Here's how the part is built. I have some questions about the finished solid (model axes, mm). A direction names the side the tool comes from. Round coordinates to 2 decimals unless told otherwise and drop trailing zeros. Order: outer loops, then holes, each group sorted by start corner. A loop starts at its lowest first (then second) coordinate and runs counter-clockwise, first axis right, second up.
```python
from build123d import *

# Parameters (mm, degrees)
F1_DEPTH = 15
F2_W     = 81.2403840464
F2_H     = 7.5
F3_DEPTH = 15
F4_DEPTH = 0.62
F5_DEPTH = 0.62


with BuildPart() as f1:
    # F0 (on Top) → F1 (new body)
    with BuildSketch(Plane.XY):
        with BuildLine():
            Line((-8.2947787642, 47.5), (-8.2947787642, 0))
            Line((-8.2947787642, 0), (20.2052212358, 0))
            ThreePointArc((20.2052212358, 0), (26.7052212358, 6.5), (33.2052212358, 0))
            Line((33.2052212358, 0), (54.2052212358, 0))
            ThreePointArc((54.2052212358, 0), (48.4723420076, 26.148498987), (32.3254132589, 47.5))
            Line((32.3254132589, 47.5), (-8.2947787642, 47.5))
        make_face()
        with BuildLine():
            Line((20.2052212358, 0), (-8.2947787642, 0))
            Line((-8.2947787642, 0), (-8.2947787642, -62.5))
            ThreePointArc((-8.2947787642, -62.5), (35.8993950599, -44.1941738242), (54.2052212358, 0))
            Line((54.2052212358, 0), (33.2052212358, 0))
            ThreePointArc((33.2052212358, 0), (26.7052212358, -6.5), (20.2052212358, 0))
        make_face()
        with BuildLine():
            Line((-8.2947787642, 0), (-36.7947787642, 0))
            ThreePointArc((-36.7947787642, 0), (-43.2947787642, -6.5), (-49.7947787642, 0))
            Line((-49.7947787642, 0), (-70.7947787642, 0))
            ThreePointArc((-70.7947787642, 0), (-52.4889525884, -44.1941738242), (-8.2947787642, -62.5))
            Line((-8.2947787642, -62.5), (-8.2947787642, 0))
        make_face()
        with BuildLine():
            ThreePointArc((-49.7947787642, 0), (-43.2947787642, 6.5), (-36.7947787642, 0))
            Line((-36.7947787642, 0), (-8.2947787642, 0))
            Line((-8.2947787642, 0), (-8.2947787642, 47.5))
            Line((-8.2947787642, 47.5), (-48.9149707874, 47.5))
            ThreePointArc((-48.9149707874, 47.5), (-65.0618995361, 26.148498987), (-70.7947787642, 0))
            Line((-70.7947787642, 0), (-49.7947787642, 0))
        make_face()
    extrude(amount=F1_DEPTH)

    # F2 (on face) → F3 (cut)
    with BuildSketch(Plane(origin=(0, 47.5, 0), x_dir=(-1, 0, 0), z_dir=(0, 1, 0))):
        with Locations((8.2947787642, 3.75)):
            Rectangle(F2_W, F2_H)
    extrude(amount=-F3_DEPTH, mode=Mode.SUBTRACT)

    # F4 (add): a face of the model
    f4_faces = [f1.faces().sort_by_distance(p)[0] for p in [
        (-48.9149707874, 40, 3.75),
    ]]
    extrude(f4_faces, amount=F4_DEPTH)

    # F5 (add): a face of the model
    f5_faces = [f1.faces().sort_by_distance(p)[0] for p in [
        (32.3254132589, 40, 3.75),
    ]]
    extrude(f5_faces, amount=F5_DEPTH)


solid = f1.part
```
1) For faces 1 (the flat face through (-7, -7, 0)), 2 (the flat face through (-48.295, 40, 4)), which set-ups out of +Z, -Z, +X, -X, +Y, -Y let a thin tool reach every point of the face, with its end or its side?
2) If we section it at C-C (x = 12): Write out the boundary of the cut face in (y, z), plus the area to 3 significant figures.
3) If we section it at D-D (z = 4): Write out the boundary of the cut face in (x, y).
4) If we section it at B-B (y = -3.5): Write out the boundary of the cut face in (x, z).
5) I'm going to push flat-ended pins straight in: pin 1 (16.5 mm diameter, centred on x = -0.5, y = 41.5, fed in from -Z); pin 2 (1.5 mm diameter, centred on y = 11.5, z = 3.5, fed in from -X); pin 3 (11.5 mm diameter, centred on x = -43.29, y = 0, fed in from +Z); pin 4 (2 mm diameter, centred on y = -50.5, z = 2, fed in from +X). Where does each tip first touch, or does it pass through?
6) We'd pull the mould along X, two halves only. Please class faces 3 (the flat face through (-8, 32.5, 4)), 4 (the flat face through (-8, 47.5, 12)): +X half, -X half, draft (parallel to the pull), parting line (faces both ways), or undercut.
7) I need wall thicknesses on line 1 (Y direction, x = 27, z = 14); line 2 (Y direction, x = -41, z = 8); line 3 (Z direction, x = -15, y = 36.5). Which ranges of each line are inside material? Lowest first, please.
8) If we section it at A-A (z = 10.75): Write out the boundary of the cut face in (x, y), plus the area to 3 significant figures.
Solutions:
1. face 1: -Z, +X, -X, +Y, -Y
1. face 2: -Z, +Y
2. outline: (-59.11, 0) - (32.5, 0) - (32.5, 7.5) - (47.5, 7.5) - (47.5, 15) - (-59.11, 15) - close
2. area: 1,490 mm2
3. outline: (-48.91, 47.5) arc R62.5 ccw (long way) to (32.33, 47.5) - (31.71, 47.5) - (31.71, 32.5) - (-48.29, 32.5) - (-48.29, 47.5) - close; hole circle Ø13 at (-43.29, 0); hole circle Ø13 at (26.71, 0)
4. outline: (-70.7, 0) - (-48.77, 0) - (-48.77, 15) - (-70.7, 15) - close; (-37.82, 0) - (21.23, 0) - (21.23, 15) - (-37.82, 15) - close; (32.18, 0) - (54.11, 0) - (54.11, 15) - (32.18, 15) - close
5. pin 1: stops at z = 7.5
5. pin 2: stops at x = -69.86
5. pin 3: passes through
5. pin 4: stops at x = 29.86
6. face 3: undercut
6. face 4: draft
7. line 1: y = -51.58 to -6.49, 6.49 to 47.5
7. line 2: y = -53.26 to -6.08, 6.08 to 47.5
7. line 3: z = 7.5 to 15
8. outline: (-48.91, 47.5) arc R62.5 ccw (long way) to (32.33, 47.5) - close; hole circle Ø13 at (-43.29, 0); hole circle Ø13 at (26.71, 0)
8. area: 11,200 mm2
